```python
from build123d import *

# Parameters (mm, degrees)
F0_R     = 20
F1_DEPTH = 5
F2_R     = 2.5
F3_R     = 2.5
F4_DEPTH = 25
F5_R     = 6
F6_DEPTH = 2


# Not quite as in the source:
# - a feature names something its author has since deleted; it is built from what else it names


with BuildPart() as f1:
    # F0 (on Top) → F1 (new body)
    with BuildSketch(Plane.XY):
        Circle(F0_R)
    extrude(amount=F1_DEPTH)

    # F2
    f2_edges = [f1.edges().sort_by_distance(p)[0] for p in [
        (-20, 0, 5),
    ]]
    fillet(f2_edges, radius=F2_R)

    # F3 (on Top) → F4 (cut)
    with BuildSketch(Plane.XY):
        with BuildLine():
            ThreePointArc((2.5, 5), (-1.767766953, 6.767766953), (0, 2.5))
            ThreePointArc((0, 2.5), (1.767766953, 3.232233047), (2.5, 5))
        make_face()
        with Locations((-5, 0)):
            Circle(F3_R)
        with BuildLine():
            ThreePointArc((2.5, -5), (1.767766953, -3.232233047), (0, -2.5))
            ThreePointArc((0, -2.5), (-1.767766953, -6.767766953), (2.5, -5))
        make_face()
        with BuildLine():
            ThreePointArc((7.5, 0), (5, 2.5), (2.5, 0))
            ThreePointArc((2.5, 0), (5, -2.5), (7.5, 0))
        make_face()
    extrude(amount=F4_DEPTH, mode=Mode.SUBTRACT)

    # F5 (on Top) → F6 (cut)
    with BuildSketch(Plane.XY):
        Circle(F5_R)
    extrude(amount=F6_DEPTH, mode=Mode.SUBTRACT)


solid = f1.part
```
Verification items for the finished model (mm, model axes). A direction names the side the tool comes from. Coordinates: 2 decimals unless noted, no trailing zeros. Order: outer loops, then holes, each group sorted by start corner. A loop starts at its lowest first (then second) coordinate and runs counter-clockwise, first axis right, second up. Notation, with made-up numbers: (-32.5, 34) -> (13.5, 34) arc R35 ccw to (13.5, 72) -> close; hole circle Ø1 at (-15, 81). An arc over 180 degrees is marked (long way). Put each result on its own line as item: value. Start each with the question number.
1) Material ranges on L1, parallel to Y at x = 0, z = 2.4; L2, parallel to Y at x = 0, z = 3.95; L3, parallel to Z at x = 1, y = -2, recorded low to high.
2) Cross-section at C-C (z = 3.45). Enter the section's corners in (x, y), plus the area to 3 significant figures.
3) Go/stop test with flat-tipped pins: pin 1 (4.5 mm diameter, centred on x = 0, y = 5, fed in from +Z); pin 2 (1.5 mm diameter, centred on x = -11, z = 4, fed in from -Y); pin 3 (1.5 mm diameter, centred on y = -3, z = 1, fed in from -X). Record where each tip stops, or that it passes through.
4) Cross-section at A-A (z = 1.2). Enter the section's corners in (x, y) (3 decimals).
5) Release check for a two-part mould opening along Y. For faces 1 (the cylindrical face through (-4.336, -19.524, 1.232)), 2 (the flat face through (0, 0, 2)), 3 (the flat face through (0, 0, 5)) record: pulls with the +Y half, pulls with the -Y half, needs draft (parallel to the pull), parting line crosses it, or undercut.
6) Tool access check on faces 4 (the cylindrical face through (7, 1.5, 3)), 5 (the cylindrical face through (4.264, 4.221, 0.986)). Record the directions out of +Z, -Z, +X, -X, +Y, -Y that give a thin tool (end or side, any length) a straight path to the whole face; none if there is none.
7) Cross-section at B-B (y = 0). Enter the section's corners in (x, z), plus the area to 3 significant figures.
Geometry check:
1. L1: y = -20 to -7.5, -2.5 to 2.5, 7.5 to 20
1. L2: y = -19.54 to -7.5, -2.5 to 2.5, 7.5 to 19.54
1. L3: z = 2 to 5
2. outline: circle Ø39.62 at (0, 0); hole circle Ø5 at (-5, 0); hole circle Ø5 at (0, -5); hole circle Ø5 at (0, 5); hole circle Ø5 at (5, 0)
2. area: 1,150 mm^2
3. pin 1: passes through
3. pin 2: stops at y = -16.81
3. pin 3: stops at x = -19.87
4. outline: circle Ø40 at (0, 0); hole (-5.475, -2.454) arc R6 ccw to (-2.454, -5.475) arc R2.5 ccw to (2.454, -5.475) arc R6 ccw to (5.475, -2.454) arc R2.5 ccw to (5.475, 2.454) arc R6 ccw to (2.454, 5.475) arc R2.5 ccw to (-2.454, 5.475) arc R6 ccw to (-5.475, 2.454) arc R2.5 ccw to start
5. face 1: parting line crosses it
5. face 2: undercut
5. face 3: needs draft
6. face 4: +Z, -Z
6. face 5: -Z
7. outline: (-20, 0) -> (-7.5, 0) -> (-7.5, 5) -> (-17.5, 5) arc R2.5 ccw to (-20, 2.5) -> close; (-2.5, 2) -> (2.5, 2) -> (2.5, 5) -> (-2.5, 5) -> close; (7.5, 0) -> (20, 0) -> (20, 2.5) arc R2.5 ccw to (17.5, 5) -> (7.5, 5) -> close
7. area: 137 mm^2
